Print and shaded views of the part. All mm, measured from the part's lowest x, y and z. Give positions to 0.01 mm unless a question says otherwise; leave off trailing zeros. Loops run counter-clockwise (first coordinate to the right, second up) from the corner with the lowest first, then second, coordinate; pieces in that order, holes last. Notation, with made-up numbers: M 44,79.25 L 59,79.25 A23 cw 59,96.25 Z; hole C 46,81 d9. An arc over 180 degrees is marked long. Answer in a Markdown table with one row per item.
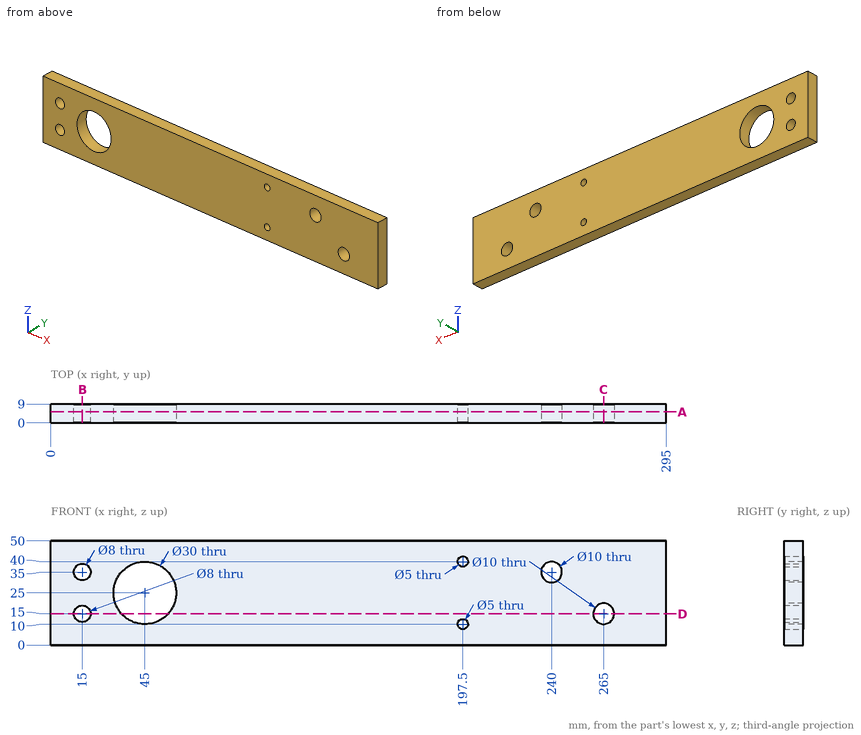
(1) Flat gauge pin, fed straight in: P1, Ø13, axis at x = 15, z = 35, coming from the +Y side. Where does the tip first touch, or does it go through?
Established:
| item | result |
|---|---|
| P1 | stops at y = 9 |
(2) Saw through at A-A, the plane y = 5.25. Give the cut face in (x, z).
Established:
| item | result |
|---|---|
| outline | M 0,0 L 295,0 L 295,50 L 0,50 Z; hole C 15,15 d8; hole C 15,35 d8; hole C 45,25 d30; hole C 197.5,10 d5; hole C 197.5,40 d5; hole C 240,35 d10; hole C 265,15 d10 |
(3) Saw through at D-D, the plane z = 15. Give the cut face in (x, y), and give its area (3 significant figures).
Established:
| item | result |
|---|---|
| outline | M 0,0 L 11,0 L 11,9 L 0,9 Z; M 19,0 L 33.82,0 L 33.82,9 L 19,9 Z; M 56.18,0 L 260,0 L 260,9 L 56.18,9 Z; M 270,0 L 295,0 L 295,9 L 270,9 Z |
| area | 2,290 mm2 |
(4) Saw through at B-B, the plane x = 15. Give the cut face in (y, z).
Established:
| item | result |
|---|---|
| outline | M 0,0 L 9,0 L 9,11 L 0,11 Z; M 0,19 L 9,19 L 9,31 L 0,31 Z; M 0,39 L 9,39 L 9,50 L 0,50 Z |
(5) Wall check: L1, parallel to Z at x = 15, y = 4.5; L2, parallel to Z at x = 197.5, y = 3.25; L3, parallel to Z at x = 265, y = 4.25. Give the ranges that are in metal, low to high.
Established:
| item | result |
|---|---|
| L1 | z = 0 to 11, 19 to 31, 39 to 50 |
| L2 | z = 0 to 7.5, 12.5 to 37.5, 42.5 to 50 |
| L3 | z = 0 to 10, 20 to 50 |
(6) Saw through at C-C, the plane x = 265. Give the cut face in (y, z), and give its area (3 significant figures).
Established:
| item | result |
|---|---|
| outline | M 0,0 L 9,0 L 9,10 L 0,10 Z; M 0,20 L 9,20 L 9,50 L 0,50 Z |
| area | 360 mm2 |
